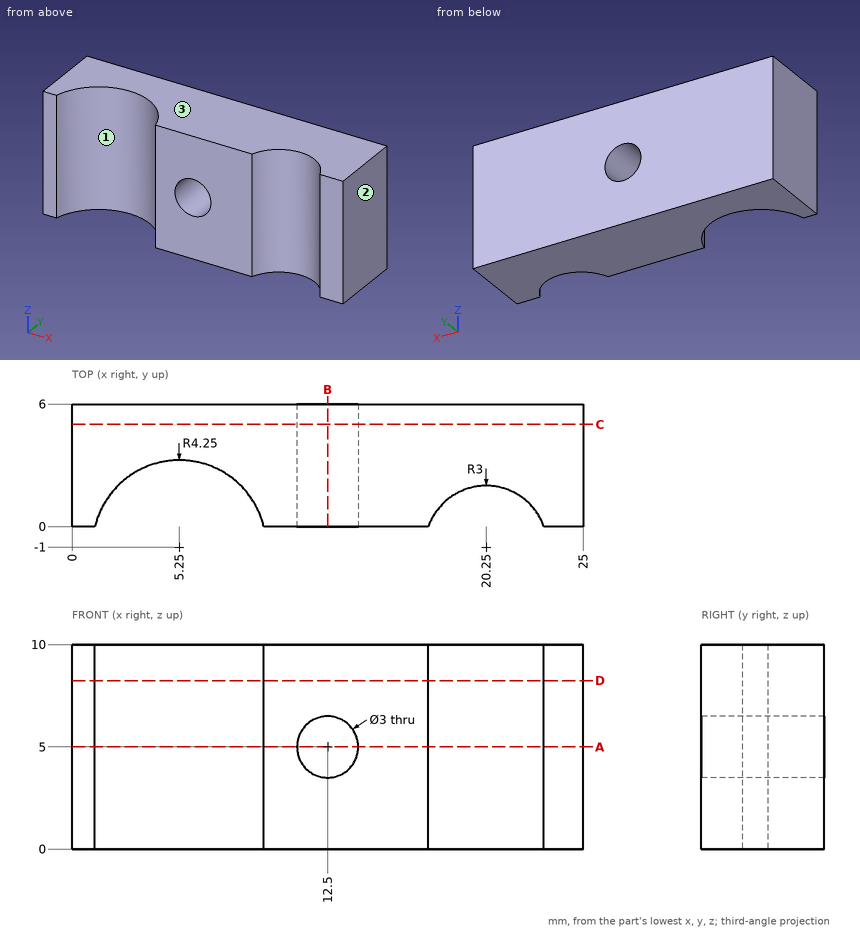
Geometry check sheet. Reference: drawing and pictorial views, mm from the part's lowest x, y, z. Coordinates: 2 decimals unless noted, no trailing zeros. Write each loop counter-clockwise with the first axis right and the second up, starting at its lowest first coordinate (ties: lowest second). Pieces come first, ordered by that corner, then holes. Notation, with made-up numbers: M -39,-12.5 L 7,-12.5 A13 ccw 7,0.5 Z; hole C -15,-38.5 d10. An arc over 180 degrees is marked long. Write item = value, one per line. Start each with the question number.
1. Sectioned sample at C-C (y = 5). Record the cut outline in (x, z), then the cut area to 3 significant figures.
2. Sectioned sample at D-D (z = 8.25). Record the cut outline in (x, y).
3. Mould release check, pull along X, two halves, no side actions. Record for the marked faces 1, 2 and 3: pulls with the +X half, pulls with the -X half, needs draft (parallel to the pull), parting line crosses it, or undercut.
4. Sectioned sample at B-B (x = 12.5). Record the cut outline in (y, z), then the cut area to 3 significant figures.
5. Sectioned sample at A-A (z = 5). Record the cut outline in (x, y), then the cut area to 3 significant figures.
6. Go/stop test with flat-tipped pins: pin 1 (1 mm diameter, centred on x = 20, z = 4.5, fed in from -Y); pin 2 (2.5 mm diameter, centred on x = 12.5, z = 5, fed in from +Y). Record where each tip stops, or that it passes through.
7. Thickness scan on probe 1 along Z at (x, y) = (12.5, 3.2); probe 2 along X at (y, z) = (1, 4.5); probe 3 along X at (y, z) = (2.15, 5). Record the ranges inside material, lowest first.
The answers:
q1.outline = M 0,0 L 25,0 L 25,10 L 0,10 Z; hole C 12.5,5 d3
q1.area = 243 mm²
q2.outline = M 0,0 L 1.12,0 A4.25 cw 9.38,0 L 17.42,0 A3 cw 23.08,0 L 25,0 L 25,6 L 0,6 Z
q3.face_1 = undercut
q3.face_2 = pulls with the +X half
q3.face_3 = needs draft
q4.outline = M 0,0 L 6,0 L 6,3.5 L 0,3.5 Z; M 0,6.5 L 6,6.5 L 6,10 L 0,10 Z
q4.area = 42.0 mm²
q5.outline = M 0,0 L 1.12,0 A4.25 cw 9.38,0 L 11,0 L 11,6 L 0,6 Z; M 14,0 L 17.42,0 A3 cw 23.08,0 L 25,0 L 25,6 L 14,6 Z
q5.area = 104 mm²
q6.pin_1 = 1.9
q6.pin_2 = through
q7.probe_1 = 0 to 3.5, 6.5 to 10
q7.probe_2 = 0 to 1.5, 9 to 11.09, 13.91 to 18.01, 22.49 to 25
q7.probe_3 = 0 to 2.4, 8.1 to 11, 14 to 25
